Solid Edge part; units mm, degrees
sketch "Sketch1" plane through (0, 0, 0) normal (0, -1, 0) x (1, 0, 0)
  line L0 (0, 19.4) -> (0, 0)
  line L1 (0, 0) -> (27, 0)
  line L2 (27, 0) -> (27, 19.4)
  line L3 (27, 19.4) -> (0, 19.4)
  line L4 (-2.4, 21.8) -> (-2.4, -2.4)
  line L5 (-2.4, -2.4) -> (29.4, -2.4)
  line L6 (29.4, -2.4) -> (29.4, 21.8)
  line L7 (29.4, 21.8) -> (-2.4, 21.8)
extrude "Protrusion1" add sketch "Sketch1" against normal blind 40
sketch "Sketch2" plane through (13.5, 20, 21.8) normal (0, 0, 1) x (-1, 0, 0)
  line L0 (4.5, -18.6) -> (4.5, -5.6)
  line L1 (4.5, -5.6) -> (10, -5.6)
  line L2 (10, -5.6) -> (10, -18.6)
  line L3 (10, -18.6) -> (4.5, -18.6)
  line L4 (-4.5, -18.6) -> (-4.5, -5.6)
  line L5 (-4.5, -5.6) -> (-10, -5.6)
  line L6 (-10, -5.6) -> (-10, -18.6)
  line L7 (-10, -18.6) -> (-4.5, -18.6)
extrude "Cutout1" cut sketch "Sketch2" against normal up to next
sketch "Sketch3" plane through (13.5, 20, -2.4) normal (0, 0, -1) x (0, 1, 0)
  line L0 (6, 5.75) -> (19, 5.75)
  line L1 (19, 5.75) -> (19, -5.75)
  line L2 (19, -5.75) -> (6, -5.75)
  line L3 (6, -5.75) -> (6, 5.75)
extrude "Cutout2" cut sketch "Sketch3" against normal up to next
sketch "Sketch4" plane through (-2.4, 20, 9.7) normal (-1, 0, 0) x (0, 0, -1)
  line L0 (-9.1, -6) -> (-9.1, 6)
  line L1 (-9.1, 6) -> (-12.1, 6)
  line L2 (-12.1, 6) -> (-12.1, -6)
  line L3 (-12.1, -6) -> (-9.1, -6)
extrude "ProtrusiónExtruida_2" add sketch "Sketch4" along normal blind 12
sketch "Sketch5" plane through (29.4, 20, 9.7) normal (1, 0, 0) x (0, 1, 0)
  line L0 (6, 12.1) -> (6, 9.1)
  line L1 (6, 9.1) -> (-6, 9.1)
  line L2 (-6, 9.1) -> (-6, 12.1)
  line L3 (-6, 12.1) -> (6, 12.1)
extrude "ProtrusiónExtruida_3" add sketch "Sketch5" along normal blind 12
fillet "Redondeo_1" radius 6 4 edges at (41.4, 14, 20.3) (41.4, 26, 20.3) (-14.4, 26, 20.3) (-14.4, 14, 20.3)
sketch "Sketch6" plane through (35.4, 20, 18.8) normal (0, 0, -1) x (-1, 0, 0)
  circle A0 centre (0, 0) radius 2
  circle A1 centre (43.8, 0) radius 2
extrude "Cutout3" cut sketch "Sketch6" against normal up to next
fillet "Redondeo_4" radius 2 6 edges at (29.4, 7, 21.8) (29.4, 33, 21.8) (-2.4, 7, 21.8) (-2.4, 33, 21.8) (-2.4, 20, -2.4) (29.4, 20, -2.4)
Source: CAD feature listing. Evaluate the final solid. Frame: model axes, mm. A direction names the side the tool comes from. Round coordinates to 2 decimals unless told otherwise and drop trailing zeros. Loops run counter-clockwise (first coordinate to the right, second up) from the corner with the lowest first, then second, coordinate; pieces in that order, holes last.
1. Section query A-A on z = 7.25. Output: boundary loops of the cut face in (x, y).
2. Section query C-C on x = 32. Output: boundary loops of the cut face in (y, z).
3. Ray query, L1, parallel to Z at x = 12.5, y = 16; L2, parallel to X at y = 18.5, z = 11.5; L3, parallel to Y at x = 35.4, z = 19.5. Return the intervals inside material, ascending.
4. Contact query for flat-ended pins moving along their axis: pin 1 (10 mm diameter, centred on y = 15.5, z = 0.5, fed in from +X); pin 2 (13 mm diameter, centred on x = 33.5, y = 22.5, fed in from -Z); pin 3 (0.7 mm diameter, centred on y = 35, z = 20, fed in from -X); pin 4 (3 mm diameter, centred on x = -8.4, y = 20, fed in from -Z). Output: stop coordinate, or through.
5. Mould query, pull axis Z, two halves, no side actions, for faces 4 (the flat face through (33, 20, 18.8)), 5 (the flat face through (0, 20, 10)), 6 (the flat face through (27, 20, 10)), 7 (the cylindrical face through (39.596, 24.289, 20.279)). Classes: released by +Z, released by -Z, zero draft, split by the parting line, or undercut.
6. Access query for faces 1 (the flat face through (-6, 20, 18.8)), 2 (the flat face through (13, 26, -1)), 3 (the flat face through (13, 20, 0)). Directions: +Z, -Z, +X, -X, +Y, -Y. A direction counts if a zero-diameter tool reaches every point of the face in a straight line with its end or side. Return the directions, or none.
7. Section query B-B on y = 13. Output: boundary loops of the cut face in (x, z), and give its area (3 significant figures).
Answers below:
1. outline: (-2.4, 0) - (0, 0) - (0, 40) - (-2.4, 40) - close; (27, 0) - (29.4, 0) - (29.4, 40) - (27, 40) - close
2. outline: (14, 18.8) - (26, 18.8) - (26, 21.8) - (14, 21.8) - close
3. L1: z = -2.4 to 0, 19.4 to 21.8
3. L2: x = -2.4 to 0, 27 to 29.4
3. L3: y = 14 to 18, 22 to 26
4. pin 1: stops at x = 29.4
4. pin 2: stops at z = -2.4
4. pin 3: stops at x = -2.4
4. pin 4: passes through
5. face 4: released by -Z
5. face 5: undercut
5. face 6: undercut
5. face 7: zero draft
6. face 1: -Z, -X, +Y, -Y
6. face 2: -Z
6. face 3: +Y, -Y
7. outline: (-2.4, -0.4) arc R2 ccw to (-0.4, -2.4) - (27.4, -2.4) arc R2 ccw to (29.4, -0.4) - (29.4, 19.8) arc R2 ccw to (27.4, 21.8) - (-0.4, 21.8) arc R2 ccw to (-2.4, 19.8) - close; hole (0, 0) - (27, 0) - (27, 19.4) - (0, 19.4) - close
7. area: 242 mm2
